```python
from build123d import *

# Parameters (mm, degrees)
F1_R        = 1.6666666667
F2_DEPTH    = 10
F3_T1_DEPTH = 46.985990025
F4_R        = 8


# Not quite as in the source:
# - a fillet or chamfer that OpenCascade refuses, or shapes differently, is made with other operations: its cross-section is extruded or revolved along the edge and cut away or added
# - a feature names something its author has since deleted; it is built from what else it names


with BuildPart() as f2:
    # F1 (on Top) → F2 (new body)
    with BuildSketch(Plane.XY):
        with BuildLine():
            ThreePointArc((7, 48.9616353347), (0, 52.3047810852), (-7, 48.9616353347))
            Line((-7, 48.9616353347), (7, 48.9616353347))
        make_face()
        with BuildLine():
            Line((7, 48.9616353347), (-7, 48.9616353347))
            Line((-7, 48.9616353347), (-7, 37.6479268357))
            ThreePointArc((-7, 37.6479268357), (0, 34.3047810852), (7, 37.6479268357))
            Line((7, 37.6479268357), (7, 48.9616353347))
        make_face()
        with Locations((0, 43.3047810852)):
            Circle(F1_R, mode=Mode.SUBTRACT)
        with BuildLine():
            Line((-7, 37.6479268357), (-7, 48.9616353347))
            ThreePointArc((-7, 48.9616353347), (-9, 43.3047810852), (-7, 37.6479268357))
        make_face()
        with BuildLine():
            ThreePointArc((9, 43.3047810852), (8.4852813742, 46.3047810852), (7, 48.9616353347))
            Line((7, 48.9616353347), (7, 37.6479268357))
            ThreePointArc((7, 37.6479268357), (8.4852813742, 40.3047810852), (9, 43.3047810852))
        make_face()
        with BuildLine():
            ThreePointArc((7, 37.6479268357), (0, 34.3047810852), (-7, 37.6479268357))
            Line((-7, 37.6479268357), (-7, -35.8969497675))
            ThreePointArc((-7, -35.8969497675), (0.0040151824, -36.6948708101), (7, -35.8293633875))
            Line((7, -35.8293633875), (7, 37.6479268357))
        make_face()
        with BuildLine():
            ThreePointArc((7, -35.8293633875), (0.0040151824, -36.6948708101), (-7, -35.8969497675))
            ThreePointArc((-7, -35.8969497675), (-23.5639927575, -25.3622297337), (-30.0136384001, -6.8217806199))
            Line((-30.0136384001, -6.8217806199), (-39.6402001052, -6.8217806199))
            Line((-39.6402001052, -6.8217806199), (-40.0136384001, -6.8217806199))
            ThreePointArc((-40.0136384001, -6.8217806199), (-0.1402001052, -46.6952189148), (39.7332381897, -6.8217806199))
            Line((39.7332381897, -6.8217806199), (29.7332381897, -6.8217806199))
            ThreePointArc((29.7332381897, -6.8217806199), (23.3728244006, -25.248934338), (7, -35.8293633875))
        make_face()
    extrude(amount=F2_DEPTH)

    # F3: chamfer of 8 on 2 edges, made by hand

    # F3_s2 → F3_t1 (cut)
    with BuildSketch(Plane.XY.offset(-18.4929950125)):
        with BuildLine():
            Line((-29.3395867315, -13.1319419656), (-37.1590781039, -6.8217806199))
            Line((-37.1590781039, -6.8217806199), (-30.0136384001, -6.8217806199))
            ThreePointArc((-30.0136384001, -6.8217806199), (-29.8322989719, -10.108356414), (-29.3395867315, -13.1319419656))
        make_face()
        with BuildLine():
            Line((36.8786778935, -6.8217806199), (29.0591865211, -13.1319419656))
            ThreePointArc((29.0591865211, -13.1319419656), (29.5518987615, -10.108356414), (29.7332381897, -6.8217806199))
            Line((29.7332381897, -6.8217806199), (36.8786778935, -6.8217806199))
        make_face()
    extrude(amount=F3_T1_DEPTH, mode=Mode.SUBTRACT)

    # F4
    f4_edges = [f2.edges().sort_by_distance(p)[0] for p in [
        (-7, -35.89695, 5),
        (7, -35.829363, 5),
    ]]
    fillet(f4_edges, radius=F4_R)


solid = f2.part
```
Check sheet for the modelled part. Datum: model origin and axes. Units: mm. A direction names the side the tool comes from. Coordinates: 2 decimals unless noted, no trailing zeros. Order: outer loops, then holes, each group sorted by start corner. A loop starts at its lowest first (then second) coordinate and runs counter-clockwise, first axis right, second up. Notation, with made-up numbers: (51.5, 50.25) -> (77.5, 50.25) arc R16 cw to (77.5, 67.25) -> close; hole circle Ø3 at (-15.5, 66.25). An arc over 180 degrees is marked (long way). Write item = value, one per line. Start each with the question number.
1) Go/stop test with flat-tipped pins: P1, Ø1.5, axis at y = 25.5, z = 4, coming from the -X side; P2, Ø3, axis at x = 17, z = 2.5, coming from the +Y side; P3, Ø3, axis at x = 22, z = 4, coming from the +Y side. Record where each tip stops, or that it passes through.
2) Cross-section at A-A (y = -11). Enter the section's corners in (x, z), then the cut area to 3 significant figures.
3) Cross-section at B-B (z = 8.5). Enter the section's corners in (x, y).
4) Material ranges on L1, parallel to X at y = -23, z = 6; L2, parallel to X at y = -12, z = 1; L3, parallel to X at y = 1, z = 8.5, recorded low to high.
5) Cross-section at D-D (y = -26). Enter the section's corners in (x, z), then the cut area to 3 significant figures.
6) Access from +Z, -Z, +X, -X, +Y, -Y to the whole of each face (thin tool, end or side, straight path). Record for faces 4 (the flat face through (7, 7, 5)), 5 (the flat face through (38, -6.822, 5)), 6 (the flat face through (0, -8, 10)), 7 (the flat face through (-39, -6.822, 5)), 8 (the cylindrical face through (-26.03, -21.73, 4.93)).
7) Cross-section at C-C (x = 0). Enter the section's corners in (y, z).
8) Mould release check, pull along X, two halves, no side actions. Record for faces 1 (the flat face through (0, -8, 0)), 2 (the cylindrical face through (-1.017, -46.686, 4.93)), 3 (the flat face through (-33.195, -10.021, 4.93)): +X half, -X half, draft (parallel to the pull), parting line (faces both ways), or undercut.
Ans:
q1.P1 = -7
q1.P2 = -29.8
q1.P3 = -25.09
q2.outline = (-39.79, 0) -> (-31.98, 0) -> (-31.98, 10) -> (-39.79, 10) -> close; (-7, 0) -> (7, 0) -> (7, 10) -> (-7, 10) -> close; (31.7, 0) -> (39.51, 0) -> (39.51, 10) -> (31.7, 10) -> close
q2.area = 296 mm²
q3.outline = (-40.01, -6.82) arc R39.87 ccw to (39.73, -6.82) -> (36.88, -6.82) -> (29.06, -13.13) arc R29.87 cw to (20.54, -28.38) arc R8 cw to (7, -22.61) -> (7, 37.65) arc R9 ccw (long way) to (-7, 37.65) -> (-7, -22.87) arc R8 cw to (-20.43, -28.74) arc R29.87 cw to (-29.34, -13.13) -> (-37.16, -6.82) -> close; hole circle Ø3.33 at (0, 43.3)
q4.L1 = -36.58 to -25.25, -7 to 7.01, 24.97 to 36.3
q4.L2 = -39.68 to -30.74, -7 to 7, 30.46 to 39.4
q4.L3 = -7 to 7
q5.outline = (-35.1, 0) -> (-23.04, 0) -> (-23.04, 10) -> (-35.1, 10) -> close; (-7.64, 0) -> (7.75, 0) -> (7.75, 10) -> (-7.64, 10) -> close; (22.76, 0) -> (34.82, 0) -> (34.82, 10) -> (22.76, 10) -> close
q5.area = 395 mm²
q6.face_4 = +Z, -Z
q6.face_5 = +Z, -Z, +X, +Y
q6.face_6 = +Z, +X, -X, +Y, -Y
q6.face_7 = +Z, -Z, -X, +Y
q6.face_8 = +Z, -Z, +Y
q7.outline = (-46.69, 0) -> (41.64, 0) -> (41.64, 10) -> (-46.69, 10) -> close; (44.97, 0) -> (52.3, 0) -> (52.3, 10) -> (44.97, 10) -> close
q8.face_1 = draft
q8.face_2 = parting line
q8.face_3 = undercut
